Autodesk Inventor part; units mm, degrees
ref_plane "YZ Plane" through (0, 0, 0) normal (1, 0, 0) x (0, 1, 0)
ref_plane "XZ Plane" through (0, 0, 0) normal (0, 1, 0) x (-1, 0, 0)
ref_plane "XY Plane" through (0, 0, 0) normal (0, 0, 1) x (1, 0, 0)
sketch "스케치1" plane through (0, 0, 0) normal (1, 0, 0) x (0, 1, 0)
  line L0 (-5.5, 4) -> (5.5, 4)
  line L1 (5.5, 4) -> (5.5, -4)
  line L2 (5.5, -4) -> (-5.5, -4)
  line L3 (-5.5, -4) -> (-5.5, 4)
  line L4 (-5.5, 4) -> (5.5, -4) construction
  line L5 (5.5, 4) -> (-5.5, -4) construction
  circle A0 centre (5.5, 0) radius 4
  circle A1 centre (5.5, 0) radius 2.1
  point P0 (0, 0)
  dimension "d0" = 8
  dimension "d1" = 11
  dimension "d2" = 4.2
extrude "돌출1" add sketch "스케치1" along normal mid plane 10.4 contours L0 A0 L2 L3 | A0 L1 A1 | L1 A1 A0
sketch "스케치2" plane through (-5.2, -5.5, 4) normal (0, 0, 1) x (1, 0, 0)
  line L0 (0.7, 17.0117) -> (9.7, 17.0117)
  line L1 (9.7, 17.0117) -> (9.7, 0.7)
  line L2 (9.7, 0.7) -> (0.7, 0.7)
  line L3 (0.7, 0.7) -> (0.7, 17.0117)
  line L4 (0.7, 17.0117) -> (9.7, 0.7) construction
  line L5 (9.7, 17.0117) -> (0.7, 0.7) construction
  line L6 (0, 0) -> (0, 11)
  line L7 (0, 0) -> (10.4, 0)
  line L8 (10.4, 11) -> (10.4, 0)
  point P0 (5.2, 5.5)
  point P1 (5.2, 8.8559)
  dimension "d5" = 0.7
  dimension "d6" = 0.7
  dimension "d7" = 0.7
extrude "돌출2" cut sketch "스케치2" against normal through all
sketch "스케치3" plane through (-4.5, -4.8, 4) normal (0, 1, 0) x (1, 0, 0)
  circle A0 centre (4.5, 4) radius 2.1
  dimension "d10" = 4.2
extrude "돌출3" cut sketch "스케치3" against normal through all
properties part number "각도엑추에이터브라켓" material "스테인리스스틸"
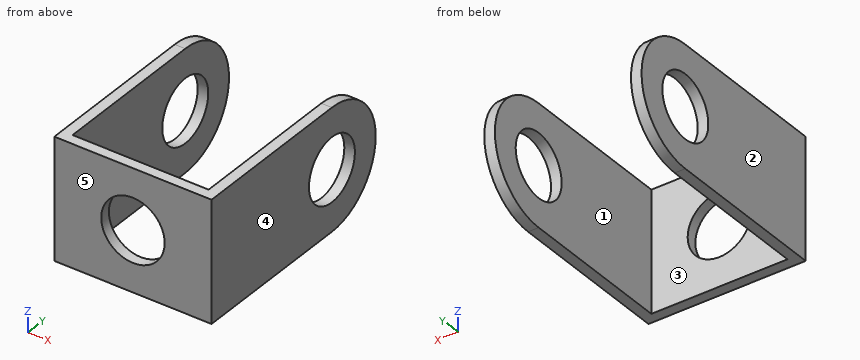
Can you work these out from the model? Positions are in its coordinate system, mm. Face numbers are marked on the shaded views. A direction names the side the tool comes from. Give positions to 0.01 mm unless a question says otherwise; leave off trailing zeros. Order: outer loops, then holes, each group sorted by start corner. A loop starts at its lowest first (then second) coordinate and runs counter-clockwise, first axis right, second up. Notation, with made-up numbers: M 8.25,-5.75 L 65.25,-5.75 A23 ccw 65.25,6.25 Z; hole C 60.5,46.25 d6. An arc over 180 degrees is marked long. Use one line per item in the form item = value.
Item 1: For the marked faces 1 and 2, which set-ups out of +Z, -Z, +X, -X, +Y, -Y let a thin tool reach every point of the face, with its end or its side?
Values follow:
face_1 = +Z, -Z, +Y
face_2 = +Z, -Z, -X, +Y, -Y
Item 2: Thinking about a two-plate mould opening in X: for the marked faces 3, 4 and 5, which applies, pulls with the +X half, pulls with the -X half, needs draft (parallel to the pull), parting line crosses it, or undercut?
Values follow:
face_3 = undercut
face_4 = pulls with the +X half
face_5 = needs draft
Item 3: If we section it at D-D, the plane y = 6.5: Write out the boundary of the cut face in (x, z).
Values follow:
outline = M -5.2,-3.87 L -4.5,-3.87 L -4.5,-1.85 L -5.2,-1.85 Z; M -5.2,1.85 L -4.5,1.85 L -4.5,3.87 L -5.2,3.87 Z; M 4.5,-3.87 L 5.2,-3.87 L 5.2,-1.85 L 4.5,-1.85 Z; M 4.5,1.85 L 5.2,1.85 L 5.2,3.87 L 4.5,3.87 Z
Item 4: If we section it at B-B, the plane z = 0: Write out the boundary of the cut face in (x, y), and give its area (3 significant figures).
Values follow:
outline = M -5.2,-5.5 L -2.1,-5.5 L -2.1,-4.8 L -4.5,-4.8 L -4.5,3.4 L -5.2,3.4 Z; M -5.2,7.6 L -4.5,7.6 L -4.5,9.5 L -5.2,9.5 Z; M 2.1,-5.5 L 5.2,-5.5 L 5.2,3.4 L 4.5,3.4 L 4.5,-4.8 L 2.1,-4.8 Z; M 4.5,7.6 L 5.2,7.6 L 5.2,9.5 L 4.5,9.5 Z
area = 18.5 mm^2
Item 5: If we section it at A-A, the plane y = -4.25: Write out the boundary of the cut face in (x, z).
Values follow:
outline = M -5.2,-4 L -4.5,-4 L -4.5,4 L -5.2,4 Z; M 4.5,-4 L 5.2,-4 L 5.2,4 L 4.5,4 Z
Item 6: If I drill on line 1 along X through (y, z) = (-5.05, 0); line 2 along Z through (x, y) = (-4.65, 5.5); line 3 along X through (y, z) = (2.5, 2), over which ranges is the centre line in solid material (lowest first)? Write a range as [from, to].
Values follow:
line_1 = [-5.2, -2.1], [2.1, 5.2]
line_2 = [-4, -2.1], [2.1, 4]
line_3 = [-5.2, -4.5], [4.5, 5.2]
Item 7: If we section it at C-C, the plane x = 0: Write out the boundary of the cut face in (y, z), and give its area (3 significant figures).
Values follow:
outline = M -5.5,-4 L -4.8,-4 L -4.8,-2.1 L -5.5,-2.1 Z; M -5.5,2.1 L -4.8,2.1 L -4.8,4 L -5.5,4 Z
area = 2.66 mm^2
Item 8: Will this pin go through, and if not, where does the flat tip stop? pin 1 Ø2.5 at (x, z) = (0, -1) entering from +Y.
Values follow:
pin_1 = -4.8
